Can you work these out from the model? Positions are in its coordinate system, mm. A direction names the side the tool comes from. Coordinates: 2 decimals unless noted, no trailing zeros. Order: outer loops, then holes, each group sorted by start corner. A loop starts at its lowest first (then second) coordinate and runs counter-clockwise, first axis right, second up. Notation, with made-up numbers: (53.5, 26.25) - (67.5, 26.25) arc R23 ccw to (67.5, 45.25) - close; hole circle Ø4 at (60.5, 50). An arc over 180 degrees is marked (long way). Use a Markdown table: item, result. Add a question column.
(1) For pin 1 Ø5 at (y, z) = (458.5, 508.5) entering from +X; pin 2 Ø6 at (y, z) = (-139, 165.5) entering from +X; pin 3 Ø12 at (x, y) = (343, 428) entering from +Z, each with a flat end and sliding along its axis, tell me the tip position at first contact or that it passes through.
(2) I want a section at A-A (y = 296). List the corners of the cut face in (x, z) for me.
(3) I want a section at B-B (z = 578.5). List the corners of the cut face in (x, y) for me.
(4) On a 3-axis mill with a long thin cutter (end or side, diameter ignored), from which of +Z, -Z, +X, -X, +Y, -Y can I reach the whole of each face in a straight line? I mean faces 1 (the flat face through (-149, -494.028, 233)), 2 (the flat face through (-551.926, 29, 685)), 3 (the flat face through (-653.526, 32, 301)). Say none if no direction works.
(5) If I drill on L1, parallel to X at y = 155, z = 336.5; L2, parallel to X at y = -43.5, z = 224; L3, parallel to Z at x = 175.5, y = -12, over which ranges is the centre line in solid material (lowest first)? Write a range as [from, to].
(6) I want a section at C-C (x = -732). List the corners of the cut face in (y, z) for me.
```python
from build123d import *

# Parameters (mm, degrees)
F0_W     = 1320.8
F0_H     = 1066.8
F1_DEPTH = 152.4
F2_W     = 1016
F2_H     = 1066.8
F3_DEPTH = 152.4
F4_W     = 711.2
F4_H     = 1066.8
F5_DEPTH = 152.4
F6_W     = 406.4
F6_H     = 1066.8
F7_DEPTH = 152.4
F9_DEPTH = 152.4


with BuildPart() as f1:
    # F0 (on Top) → F1 (new body)
    with BuildSketch(Plane.XY):
        with Locations((6.8740844727, 39.3722309107)):
            Rectangle(F0_W, F0_H)
    extrude(amount=F1_DEPTH)

    # F2 (on face) → F3 (join)
    with BuildSketch(Plane.XY.offset(152.4)):
        with Locations((-145.5259155273, 39.3722309107)):
            Rectangle(F2_W, F2_H)
    extrude(amount=F3_DEPTH)

    # F4 (on face) → F5 (join)
    with BuildSketch(Plane.XY.offset(304.8)):
        with Locations((-297.9259155273, 39.3722309107)):
            Rectangle(F4_W, F4_H)
    extrude(amount=F5_DEPTH)

    # F6 (on face) → F7 (join)
    with BuildSketch(Plane.XY.offset(457.2)):
        with Locations((-450.3259155273, 39.3722309107)):
            Rectangle(F6_W, F6_H)
    extrude(amount=F7_DEPTH)

    # F8 (on face) → F9 (join)
    with BuildSketch(Plane.XY.offset(609.6)):
        Polygon((-551.9259155273, -499.3119239807), (-551.9259155273, 572.7722309107), (-653.5259155273, 572.7722309107), (-856.7259155273, 572.7722309107), (-856.7259155273, -499.3119239807), align=None)
    extrude(amount=F9_DEPTH)


solid = f1.part
```
Answers follow:
| question | item | result |
|---|---|---|
| 1 | pin 1 | stops at x = -247.13 |
| 1 | pin 2 | stops at x = 362.47 |
| 1 | pin 3 | stops at z = 304.8 |
| 2 | outline | (-856.73, 609.6) - (-653.53, 609.6) - (-653.53, 0) - (667.27, 0) - (667.27, 152.4) - (362.47, 152.4) - (362.47, 304.8) - (57.67, 304.8) - (57.67, 457.2) - (-247.13, 457.2) - (-247.13, 609.6) - (-551.93, 609.6) - (-551.93, 762) - (-856.73, 762) - close |
| 3 | outline | (-653.53, -494.03) - (-247.13, -494.03) - (-247.13, 572.77) - (-653.53, 572.77) - close |
| 4 | face 1 | -Z, +X, -X, -Y |
| 4 | face 2 | +Z, +X, +Y, -Y |
| 4 | face 3 | -Z, -X, +Y, -Y |
| 5 | L1 | x = [-653.53, 57.67] |
| 5 | L2 | x = [-653.53, 362.47] |
| 5 | L3 | z = [0, 304.8] |
| 6 | outline | (-499.31, 609.6) - (572.77, 609.6) - (572.77, 762) - (-499.31, 762) - close |
